CAD build for the part. Positions are in the model's coordinates, mm. Coordinates: 2 decimals unless noted, no trailing zeros. Write each loop counter-clockwise with the first axis right and the second up, starting at its lowest first coordinate (ties: lowest second). Pieces come first, ordered by that corner, then holes. Notation, with made-up numbers: (1.25, -28.5) -> (34.25, -28.5) arc R18 ccw to (34.25, -12.5) -> close; hole circle Ø2 at (-27, 87.25). An arc over 180 degrees is marked (long way). Answer as CSV lines item,"result".
```python
from build123d import *

# Parameters (mm, degrees)
F1_DEPTH = 5
F3_DEPTH = 5


with BuildPart() as f1:
    # F0 (on Front) → F1 (new body)
    with BuildSketch(Plane.XZ):
        with BuildLine():
            ThreePointArc((-22.0468155789, -24.7666841827), (-6.6104134528, -16.4288071016), (-0.4543593565, 0))
            ThreePointArc((-0.4543593565, 0), (-39.618976734, 20.6000877316), (-34.4034485204, -23.3433888529))
            ThreePointArc((-34.4034485204, -23.3433888529), (-34.13988042, -23.4403115833), (-33.876793996, -23.5385342522))
            ThreePointArc((-33.876793996, -23.5385342522), (-28.0359035944, -24.8663553692), (-22.0468155789, -24.7666841827))
        make_face()
        with BuildLine():
            ThreePointArc((-4.6974495608, 0), (-13.4479875789, -16.9321097623), (-32.3216329124, -19.5880029144))
            ThreePointArc((-32.3216329124, -19.5880029144), (-32.7996241433, -19.4138195489), (-33.2732030007, -19.2279741089))
            ThreePointArc((-33.2732030007, -19.2279741089), (-37.0421605292, 17.2212708081), (-4.6974495608, 0))
        make_face(mode=Mode.SUBTRACT)
        with BuildLine():
            ThreePointArc((50.4543593565, 0), (25.4543593565, 25), (0.4543593565, 0))
            ThreePointArc((0.4543593565, 0), (6.4867521845, -16.2858797174), (21.67274961, -24.7123335144))
            ThreePointArc((21.67274961, -24.7123335144), (27.8478432396, -24.8851609378), (33.876793996, -23.5385342522))
            ThreePointArc((33.876793996, -23.5385342522), (34.13988042, -23.4403115833), (34.4034485204, -23.3433888529))
            ThreePointArc((34.4034485204, -23.3433888529), (46.0544470881, -14.1646173775), (50.4543593565, 0))
        make_face()
        with BuildLine():
            ThreePointArc((34.4034485204, -18.7286707324), (32.5837256191, -19.4941386308), (30.6995126262, -20.0832684452))
            ThreePointArc((30.6995126262, -20.0832684452), (9.0269055436, 12.6881072462), (46.2112691521, 0))
            ThreePointArc((46.2112691521, 0), (43.0129005942, -11.0700918636), (34.4034485204, -18.7286707324))
        make_face(mode=Mode.SUBTRACT)
        with BuildLine():
            ThreePointArc((0, -49.6637113392), (-9.2528617859, -35.6473438574), (-22.0468155789, -24.7666841827))
            ThreePointArc((-22.0468155789, -24.7666841827), (-28.0359035944, -24.8663553692), (-33.876793996, -23.5385342522))
            ThreePointArc((-33.876793996, -23.5385342522), (-12.9903930203, -37.2598807121), (0, -58.6085758378))
            Line((0, -58.6085758378), (0, -49.6637113392))
        make_face()
        with BuildLine():
            ThreePointArc((21.67274961, -24.7123335144), (8.9955723313, -35.5891026648), (0, -49.6637113392))
            Line((0, -49.6637113392), (0, -58.6085758378))
            ThreePointArc((0, -58.6085758378), (12.9903930203, -37.2598807121), (33.876793996, -23.5385342522))
            ThreePointArc((33.876793996, -23.5385342522), (27.8478432396, -24.8851609378), (21.67274961, -24.7123335144))
        make_face()
    extrude(amount=F1_DEPTH)

    # F2 (on face) → F3 (join)
    with BuildSketch(Plane.XZ.offset(5)):
        with BuildLine():
            Line((0, 75.4342153668), (-44.5349970754, 16.1533050563))
            ThreePointArc((-44.5349970754, 16.1533050563), (-40.3802571517, 20.0553627493), (-35.4496590764, 22.9149292713))
            Line((-35.4496590764, 22.9149292713), (0, 70.1022695262))
            Line((0, 70.1022695262), (35.4496590764, 22.9149292713))
            ThreePointArc((35.4496590764, 22.9149292713), (40.3802571517, 20.0553627493), (44.5349970754, 16.1533050563))
            Line((44.5349970754, 16.1533050563), (0, 75.4342153668))
        make_face()
    extrude(amount=-F3_DEPTH)


solid = f1.part
```
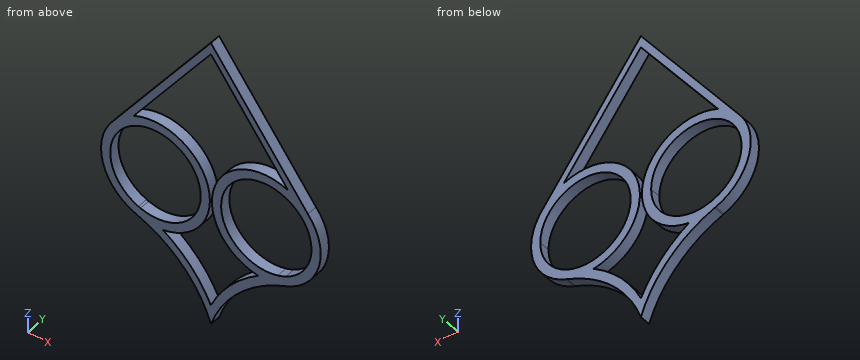
Item 1: Wall check: line 1 (X direction, y = -1, z = 1); line 2 (Z direction, x = -20, y = -2.7); line 3 (Z direction, x = 31.5, y = -1.85). Give the ranges that are in metal, low to high. Write a range as from..to.
Answer below:
line 1,"x = -50.43..-46.19, -4.72..-0.47, 0.47..4.72, 46.19..50.43"
line 2,"z = -31.1..-26.12, -24.4..-20.03, 20.03..24.4, 43.48..48.81"
line 3,"z = -24.49..-19.86, 19.86..24.26, 28.17..33.5"
Item 2: Flat gauge pins, fed straight in: pin 1 (1 mm diameter, centred on x = 19.5, y = -2, fed in from +Z); pin 2 (1.5 mm diameter, centred on x = -21, y = -2.5, fed in from +Z); pin 3 (1.5 mm diameter, centred on x = -19, y = -4.5, fed in from -Z); pin 4 (25 mm diameter, centred on x = 25.45, z = 0, fed in from -Y). Where does each tip first touch, or does it go through?
Answer below:
pin 1,"stops at z = 50.14"
pin 2,"stops at z = 48.48"
pin 3,"stops at z = -32.46"
pin 4,"passes through"
Item 3: Saw through at B-B on z = 2. Give the cut face in (x, y).
Answer below:
outline,"(-50.37, -5) -> (-46.11, -5) -> (-46.11, 0) -> (-50.37, 0) -> close; (-4.79, -5) -> (-0.53, -5) -> (-0.53, 0) -> (-4.79, 0) -> close; (0.53, -5) -> (4.79, -5) -> (4.79, 0) -> (0.53, 0) -> close; (46.11, -5) -> (50.37, -5) -> (50.37, 0) -> (46.11, 0) -> close"
Item 4: Saw through at C-C on z = -46.5. Give the cut face in (x, y).
Answer below:
outline,"(-5.75, -5) -> (-1.61, -5) -> (-1.61, 0) -> (-5.75, 0) -> close; (1.54, -5) -> (5.75, -5) -> (5.75, 0) -> (1.54, 0) -> close"
Item 5: Saw through at A-A on y = -0.8. Give the cut face in (x, z) (3 decimals).
Answer below:
outline,"(-44.535, 16.153) arc R25 ccw to (-34.403, -23.343) arc R56.886 cw to (0, -58.609) arc R56.886 cw to (34.403, -23.343) arc R25 ccw to (44.535, 16.153) -> (0, 75.434) -> close; hole circle Ø41.514 at (-25.454, 0); hole (-35.45, 22.915) arc R25 cw (long way) to (-22.047, -24.767) arc R59.636 cw to (0, -49.664) arc R57.216 cw to (21.673, -24.712) arc R25 cw (long way) to (35.45, 22.915) -> (0, 70.102) -> close; hole circle Ø41.514 at (25.454, 0)"
Item 6: Saw through at D-D on x = 32.5. Give the cut face in (y, z).
Answer below:
outline,"(-5, -24.08) -> (0, -24.08) -> (0, -19.52) -> (-5, -19.52) -> close; (-5, 19.52) -> (0, 19.52) -> (0, 23.99) -> (-5, 23.99) -> close; (-5, 26.84) -> (0, 26.84) -> (0, 32.17) -> (-5, 32.17) -> close"
